Autodesk Fusion 360 part; units mm, degrees
sketch "Sketch1" plane through (0, 0, 0) normal (0, 0, 1) x (1, 0, 0)
  circle A0 centre (0, 0) radius 3.1
  dimension "d3" = 6.2
extrude "Extrude1" add sketch "Sketch1" along normal blind 80
sketch "Sketch3" plane through (0, 0, 0) normal (0, 1, 0) x (1, 0, 0)
  line L0 (-1.4286, -3) -> (1.5714, -3)
  line L1 (1.5714, -3) -> (1.5714, -8)
  line L2 (1.5714, -8) -> (-1.4286, -8)
  line L3 (-1.4286, -8) -> (-1.4286, -3)
  line L4 (-1.4286, -77) -> (1.5714, -77)
  line L5 (1.5714, -77) -> (1.5714, -72)
  line L6 (1.5714, -72) -> (-1.4286, -72)
  line L7 (-1.4286, -72) -> (-1.4286, -77)
  line L8 (-3.1, -80) -> (3.1, -80)
  dimension "d9" = 3
  dimension "d10" = 5
  dimension "d11" = 3
  dimension "d12" = 5
  dimension "d18" = 3
  dimension "d19" = 3
extrude "Extrude2" cut sketch "Sketch3" along normal mid plane 200 contours L4 L5 L6 L7
extrude "Extrude3" cut sketch "Sketch3" along normal mid plane 200 contours L0 L1 L2 L3
equation "dowel_pin_radius = 3.10 mm"
equation "length = 80 mm"
equation "d3 = dowel_pin_radius * 2"
equation "d4 = length"
equation "hole_distance = 3 mm"
equation "hole_width = 3 mm"
equation "hole_height = 5 mm"
equation "d9 = hole_width"
equation "d10 = hole_height"
equation "d11 = hole_width"
equation "d12 = hole_height"
equation "extra = 100 mm"
equation "d14 = extra"
equation "d16 = extra"
equation "d18 = hole_distance"
equation "d19 = hole_distance"
The model under review builds one solid part; all positions refer to its coordinate system, in mm. A direction names the side the tool comes from. Coordinates: 2 decimals unless noted, no trailing zeros. Write each loop counter-clockwise with the first axis right and the second up, starting at its lowest first coordinate (ties: lowest second). Pieces come first, ordered by that corner, then holes. Notation, with made-up numbers: (68, 41.25) -> (73, 41.25) arc R23 cw to (73, 73.25) -> close; hole circle Ø7 at (22.5, 31.25). An arc over 180 degrees is marked (long way). One line per item, written item: value. Start each with the question number.
Q1. To check wall thickness, follow probe 1 along Z at (x, y) = (-1, 1.25); probe 2 along Y at (x, z) = (-0.25, 40.5); probe 3 along X at (y, z) = (1, 4). State the ranges of each line that lie inside material, in increasing order.
Q2. Add section C-C, the plane z = 57. Give the boundary of the cut face in (x, y), then the cut area to 3 significant figures.
Q3. For faces 1 (the face through (0, 0, 80)), 2 (the face through (0, 0, 72)), list the 3-axis set-ups (+Z, -Z, +X, -X, +Y, -Y) from which the entire face can be reached by the end or side of a thin tool; tool diameter is ignored.
Q4. Add section A-A, the plane y = 0. Give the boundary of the cut face in (x, z).
Q5. Clearance check with flat-ended pins moving along their axes: P1, Ø2.5, axis at y = 0.5, z = 73.5, coming from the +X side; P2, Ø1, axis at y = 1, z = 69, coming from the -X side. State where each tip first meets the part, or that it passes through.
Q6. Add section B-B, the plane x = 0. Give the boundary of the cut face in (y, z).
Q7. The part is to be moulded in two halves that separate along X. For faces 3 (the face through (0, 0, 0)), 4 (the face through (-0.404, -3.074, 39.44)), 5 (the face through (0, 0, 3)), say which applies: +X half, -X half, draft (parallel to the pull), parting line (faces both ways), or undercut.
Response:
1. probe 1: 0 to 3, 8 to 72, 77 to 80
1. probe 2: -3.09 to 3.09
1. probe 3: -2.93 to -1.43, 1.57 to 2.93
2. outline: circle Ø6.2 at (0, 0)
2. area: 30.2 mm²
3. face 1: +Z, +X, -X, +Y, -Y
3. face 2: +Y, -Y
4. outline: (-3.1, 0) -> (3.1, 0) -> (3.1, 80) -> (-3.1, 80) -> close; hole (-1.43, 3) -> (1.57, 3) -> (1.57, 8) -> (-1.43, 8) -> close; hole (-1.43, 72) -> (1.57, 72) -> (1.57, 77) -> (-1.43, 77) -> close
5. P1: x = 3.1
5. P2: x = -3.06
6. outline: (-3.1, 0) -> (3.1, 0) -> (3.1, 3) -> (-3.1, 3) -> close; (-3.1, 8) -> (3.1, 8) -> (3.1, 72) -> (-3.1, 72) -> close; (-3.1, 77) -> (3.1, 77) -> (3.1, 80) -> (-3.1, 80) -> close
7. face 3: draft
7. face 4: parting line
7. face 5: undercut
